Design review of the part built by this model. Coordinates are the model's own, in mm. A direction names the side the tool comes from. Give positions to 0.01 mm unless a question says otherwise; leave off trailing zeros. Loops run counter-clockwise (first coordinate to the right, second up) from the corner with the lowest first, then second, coordinate; pieces in that order, holes last. Notation, with made-up numbers: (22.5, 33.25) - (73.5, 33.25) arc R8 cw to (73.5, 39.25) - close; hole circle Ø4 at (46.25, 44.25). An arc over 180 degrees is marked (long way). Put each result on its own line as item: value. Start each with the question number.
Solid Edge part; units mm, degrees
sketch "Sketch1" plane through (0, 0, 0) normal (0, 0, 1) x (1, 0, 0)
  line L0 (1, 2.5) -> (1.4606, 11.2)
  line L1 (0.85, 11.2) -> (1.4606, 11.2)
  line L2 (0.85, 13.7) -> (0.85, 11.2)
  line L3 (0.85, 13.7) -> (8.85, 13.7)
  line L4 (8.85, 11.2) -> (8.85, 13.7)
  line L5 (8.85, 11.2) -> (8.2394, 11.2)
  line L6 (8.7, 2.5) -> (8.2394, 11.2)
  line L7 (9.7, 2.5) -> (8.7, 2.5)
  line L8 (9.7, 0) -> (9.7, 2.5)
  line L9 (0, 0) -> (9.7, 0)
  line L10 (0, 2.5) -> (0, 0)
  line L11 (0, 2.5) -> (1, 2.5)
extrude "Protrusion1" add sketch "Sketch1" along normal up to vertex (8.1 mm away)
sketch "Sketch2" plane through (0, 0, 0) normal (1, 0, 0) x (0, 1, 0)
  line L0 (11.2, 0) -> (13.7, 0)
  line L1 (13.7, 0) -> (13.7, 8.1)
  line L2 (13.7, 8.1) -> (11.2, 8.1)
  arc A0 (2.5, 8.1) -> (11.2, 8.1) centre (6.85, 17.0612) ccw
  line L3 (2.5, 8.1) -> (0, 8.1)
  line L4 (0, 8.1) -> (0, 0)
  line L5 (0, 0) -> (2.5, 0)
  arc A1 (2.5, 0) -> (11.2, 0) centre (6.85, -8.9613) cw
extrude "Cutout1" cut sketch "Sketch2" along normal blind 13.0896 flip side to cut
sketch "Sketch3" plane through (4.85, 10.275, 0) normal (0, 0, -1) x (-1, 0, 0)
  line L0 (1.25, -3.425) -> (0, 0.3758)
  line L1 (0, 0.3758) -> (-1.25, -3.425)
  line L2 (0, -3.425) -> (-1.25, -3.425)
  line L3 (0, -3.425) -> (1.25, -3.425)
extrude "TriangleProtrusion" add sketch "Sketch3" against normal blind 2.6122
sketch "Sketch4" plane through (4.85, 13.7, 4.05) normal (0, 1, 0) x (1, 0, 0)
  line L0 (0.8, 0.8) -> (0.8, 2.125)
  line L1 (0.8, 2.125) -> (-0.8, 2.125)
  line L2 (-0.8, 2.125) -> (-0.8, 0.8)
  line L3 (-0.8, 0.8) -> (-2.125, 0.8)
  line L4 (-2.125, 0.8) -> (-2.125, -0.8032)
  line L5 (-2.125, -0.8032) -> (-0.8, -0.8)
  line L6 (-0.8, -0.8) -> (-0.8, -2.125)
  line L7 (-0.8, -2.125) -> (0.8, -2.125)
  line L8 (0.8, -2.125) -> (0.8, -0.8)
  line L9 (0.8, -0.8) -> (2.125, -0.793)
  line L10 (2.125, -0.793) -> (2.125, 0.8)
  line L11 (2.125, 0.8) -> (0.8, 0.8)
extrude "Protrusion2" add sketch "Sketch4" along normal up to vertex (6.5 mm away)
sketch "Sketch5" plane through (4.85, 20.2, 4.05) normal (0, 1, 0) x (1, 0, 0)
  circle A0 centre (0, 0) radius 0.75
extrude "ShaftProtrusion" add sketch "Sketch5" along normal blind 45
Item 1: Consider section A-A (z = 4.05). State the section outline as (x, y) points (3 decimals), plus the area to 3 significant figures.
Item 2: For L1, parallel to Y at x = 5, z = 3; L2, parallel to Y at x = 7.75, z = 2.5; L3, parallel to X at y = 12, z = 1.5, list the stretches that pass through material, from the lowest coordinate up. Write a range as from..to.
Item 3: Machinability: for faces 4 (the flat face through (5, 17, 6.175)), 5 (the flat face through (8.473, 6.789, 3.993)), 6 (the flat face through (4.05, 17, 6)), which of the approach directions +Z, -Z, +X, -X, +Y, -Y give a long, thin tool a straight path to every point of the face, cutting with its end or side? Answer none if there is none.
Item 4: For P1, Ø5, axis at x = 3, y = 43.5, coming from the +Z side; P2, Ø0.5, axis at y = 18, z = 4.5, coming from the -X side (3 decimals); P3, Ø1.8, axis at x = 5, y = 17, coming from the +Z side (3 decimals), all flat-tipped, find the tip position at first contact; note any pin that passes through.
Item 5: Mouldability with a two-part tool opening along Y and no side actions: class faces 1 (the flat face through (1.227, 6.789, 3.993)), 2 (the flat face through (5, 0, 4)), 3 (the flat face through (0, 1, 4)) as pulls with the +Y half, pulls with the -Y half, needs draft (parallel to the pull), parting line crosses it, or undercut.
Item 6: Consider section C-C (y = 59.5). State the section outline as (x, z) points, plus the area to 3 significant figures.
Item 7: Consider section B-B (y = 18). State the section outline as (x, z) points (3 decimals).
Geometry says:
1. outline: (0, 0) - (9.7, 0) - (9.7, 2.5) - (8.7, 2.5) - (8.239, 11.2) - (8.85, 11.2) - (8.85, 13.7) - (6.975, 13.7) - (6.975, 20.2) - (5.6, 20.2) - (5.6, 65.2) - (4.1, 65.2) - (4.1, 20.2) - (2.725, 20.2) - (2.725, 13.7) - (0.85, 13.7) - (0.85, 11.2) - (1.461, 11.2) - (1, 2.5) - (0, 2.5) - close
1. area: 202 mm2
2. L1: y = 0..20.2
2. L2: y = 0..13.7
2. L3: x = 0.85..8.85
3. face 4: +Z, +X, -X, +Y
3. face 5: +Z, -Z, +X
3. face 6: +Z, -X, +Y
4. P1: stops at z = 4.8
4. P2: stops at x = 2.725
4. P3: stops at z = 6.175
5. face 1: undercut
5. face 2: pulls with the -Y half
5. face 3: needs draft
6. outline: circle Ø1.5 at (4.85, 4.05)
6. area: 1.77 mm2
7. outline: (2.725, 3.25) - (4.05, 3.25) - (4.05, 1.925) - (5.65, 1.925) - (5.65, 3.25) - (6.975, 3.25) - (6.975, 4.843) - (5.65, 4.85) - (5.65, 6.175) - (4.05, 6.175) - (4.05, 4.85) - (2.725, 4.853) - close
